Here's how the part is built. I have some questions about the finished solid (model axes, mm). A direction names the side the tool comes from. Round coordinates to 2 decimals unless told otherwise and drop trailing zeros. Loops run counter-clockwise (first coordinate to the right, second up) from the corner with the lowest first, then second, coordinate; pieces in that order, holes last. Notation, with made-up numbers: (-0.5, 9.5) - (8.5, 9.5) arc R19 cw to (8.5, 40.5) - close; hole circle Ø4 at (18, 50). An arc over 180 degrees is marked (long way). Answer as a JSON object with one key per item and string values. Group by question number.
1) Which directions (+Z, -Z, +X, -X, +Y, -Y) give clear straight access to the entire face, cutting with the end or side of a thin tool? Please do faces 5 (the face through (165, -40, 15)), 6 (the face through (80.13, -24, 0)), 7 (the face through (165, -22, -10)).
2) I want a section at D-D, the plane y = -51. Please give me the cut outline in (x, z), then the cut area to 3 significant figures.
3) I want a section at B-B, the plane y = -33. Please give me the cut outline in (x, z), then the cut area to 3 significant figures.
4) Will these pins go through, and if not, where does the flat tip stop? P1, Ø5, axis at x = 113, y = -52.5, coming from the +Z side; P2, Ø10, axis at x = 161.5, y = -26.5, coming from the -Z side; P3, Ø7, axis at y = -54, z = -8.5, coming from the -X side.
5) If we mould it in two halves opening along Y, with no side actions, what happens to faces 1 (the face through (113.06, -57.003, 0.238)), 2 (the face through (81.65, -20.7, 0.11)), 3 (the face through (123, -6, 17)), 4 (the face through (118.13, -36, 2))? For each: pulls with the +Y half, pulls with the -Y half, needs draft (parallel to the pull), parting line crosses it, or undercut.
6) I want a section at C-C, the plane z = 5. Please give me the cut outline in (x, y).
7) I want a section at A-A, the plane x = 49.5. Please give me the cut outline in (y, z).
8) If I drill on line 1 along X through (y, z) = (-21, 8); line 2 along Z through (x, y) = (40, -19.5); line 3 along X through (y, z) = (-40.5, 9), over which ranges is the centre line in solid material (lowest first)? Write a range as [from, to].
from build123d import *

# Parameters (mm, degrees)
EXTRUDE_1_DEPTH     = 17
EXTRUDE_2_DEPTH     = 20
SKETCH_2_W          = 127.5
SKETCH_2_H          = 12.22
CUT_EXTRUDE_1_DEPTH = 17
SKETCH_6_W          = 30
SKETCH_6_H          = 40
CUT_EXTRUDE_2_DEPTH = 10
SKETCH_7_W          = 30
SKETCH_7_H          = 40
CUT_EXTRUDE_3_DEPTH = 10
SKETCH_8_W          = 67
SKETCH_8_H          = 22.78
CUT_EXTRUDE_4_DEPTH = 14
CUT_EXTRUDE_6_DEPTH = 7.5
CUT_EXTRUDE_7_REACH = 192.46
CHAMFER_1_SIZE      = 1


with BuildPart() as part:
    # 스케치1 → 보스-돌출1 (new, symmetric)
    with BuildSketch(Plane.XY):
        Polygon((180, 0), (0, 0), (0, -35), (118.13, -35), (118.13, -45), (108.13, -45), (108.13, -58.95), (118.13, -55), (180, -55), align=None)
    extrude(amount=EXTRUDE_1_DEPTH, both=True)

    # 스케치1<3> → 보스-돌출2 (add, symmetric)
    with BuildSketch(Plane.XY):
        Polygon((180, 0), (127.5, 0), (118.13, 0), (118.13, -10), (118.13, -35), (118.13, -45), (118.13, -55), (180, -55), align=None)
    extrude(amount=EXTRUDE_2_DEPTH, both=True)

    # 스케치2 → 컷-돌출1 (cut, symmetric)
    with BuildSketch(Plane.XY):
        with Locations((63.75, -6.11)):
            Rectangle(SKETCH_2_W, SKETCH_2_H)
    extrude(amount=CUT_EXTRUDE_1_DEPTH, both=True, mode=Mode.SUBTRACT)

    # 스케치6 → 컷-돌출2 (cut)
    with BuildSketch(Plane.XY.offset(20)):
        with Locations((165, -20)):
            Rectangle(SKETCH_6_W, SKETCH_6_H)
    extrude(amount=-CUT_EXTRUDE_2_DEPTH, mode=Mode.SUBTRACT)

    # 스케치7 → 컷-돌출3 (cut)
    with BuildSketch(Plane(origin=(0, 0, -20), x_dir=(-1, 0, 0), z_dir=(0, 0, -1))):
        with Locations((-165, -20)):
            Rectangle(SKETCH_7_W, SKETCH_7_H)
    extrude(amount=-CUT_EXTRUDE_3_DEPTH, mode=Mode.SUBTRACT)

    # 스케치8 → 컷-돌출4 (cut, symmetric)
    with BuildSketch(Plane.XY):
        with Locations((46.63, -23.61)):
            Rectangle(SKETCH_8_W, SKETCH_8_H)
    extrude(amount=CUT_EXTRUDE_4_DEPTH, both=True, mode=Mode.SUBTRACT)

    # 스케치13 → 컷-돌출6 (cut, symmetric)
    with BuildSketch(Plane.XY):
        Polygon((80.13, -16.22), (83.13, -19.22), (80.13, -22.22), align=None)
    extrude(amount=CUT_EXTRUDE_6_DEPTH, both=True, mode=Mode.SUBTRACT)

    # 컷-돌출7: up to this face of the body (flat: up to its plane)
    cut_extrude_7_end = Plane(part.part.faces().sort_by_distance((127.5, -6.11, 0))[0])
    # 스케치14 → 컷-돌출7 (cut, up to the picked face)
    with BuildSketch(Plane(origin=(180, 0, 0), x_dir=(0, 0, -1), z_dir=(1, 0, 0)), mode=Mode.PRIVATE) as cut_extrude_7_sk1:
        with BuildLine():
            Line((-12.990381057, 0), (12.990381057, 0))
            ThreePointArc((12.990381057, 0), (0, -7.5), (-12.990381057, 0))
        make_face()
    cut_extrude_7_tool1 = split(extrude(cut_extrude_7_sk1.sketch, amount=-CUT_EXTRUDE_7_REACH, mode=Mode.PRIVATE), bisect_by=cut_extrude_7_end, keep=Keep.BOTH, mode=Mode.PRIVATE)
    add(cut_extrude_7_tool1.solids().sort_by(Axis((180, -3.075302, 0), (-1, 0, 0)))[0], mode=Mode.SUBTRACT)

    # 모따기1
    chamfer_1_edges = [part.edges().sort_by_distance(p)[0] for p in [
        (149.065, -55, -20),
        (149.065, -55, 20),
    ]]
    chamfer(chamfer_1_edges, length=CHAMFER_1_SIZE)


solid = part.part
Outcome:
{
 "1": {"face 5": "+Z, +X, +Y", "face 6": "+Y, -Y", "face 7": "-Z, +X, +Y"},
 "2": {"outline": "(108.13, -17) - (118.13, -17) - (118.13, -20) - (180, -20) - (180, 20) - (118.13, 20) - (118.13, 17) - (108.13, 17) - close", "area": "2,810 mm^2"},
 "3": {"outline": "(0, -17) - (118.13, -17) - (118.13, -20) - (150, -20) - (150, -10) - (180, -10) - (180, 10) - (150, 10) - (150, 20) - (118.13, 20) - (118.13, 17) - (0, 17) - close; hole (13.13, -14) - (80.13, -14) - (80.13, 14) - (13.13, 14) - close", "area": "4,020 mm^2"},
 "4": {"P1": "z = 17", "P2": "z = -10", "P3": "x = 108.13"},
 "5": {"face 1": "pulls with the -Y half", "face 2": "undercut", "face 3": "needs draft", "face 4": "undercut"},
 "6": {"outline": "(0, -35) - (13.13, -35) - (13.13, -12.22) - (0, -12.22) - close; (80.13, -35) - (118.13, -35) - (118.13, -45) - (108.13, -45) - (108.13, -58.95) - (118.13, -55) - (180, -55) - (180, -6.64) - (127.5, -6.64) - (127.5, -12.22) - (80.13, -12.22) - (80.13, -16.22) - (83.13, -19.22) - (80.13, -22.22) - close"},
 "7": {"outline": "(-35, -17) - (-12.22, -17) - (-12.22, -14) - (-35, -14) - close; (-35, 14) - (-12.22, 14) - (-12.22, 17) - (-35, 17) - close"},
 "8": {"line 1": "[0, 13.13], [80.13, 180]", "line 2": "[-17, -14], [14, 17]", "line 3": "[118.13, 180]"}
}
